Here's the drawing with two shaded views (mm, measured from the low corner). I have some questions. Coordinates: 2 decimals unless noted, no trailing zeros. Order: outer loops, then holes, each group sorted by start corner. A loop starts at its lowest first (then second) coordinate and runs counter-clockwise, first axis right, second up. Notation, with made-up numbers: (-1, 79.5) - (34, 79.5) arc R15 cw to (34, 91.5) - close; hole circle Ø5 at (73.25, 42). An arc over 180 degrees is marked (long way). Answer as a JSON object with one key per item and string values. Group by question number.
(1) Will these pins go through, and if not, where does the flat tip stop? P1, Ø0.9, axis at y = 5.5, z = 2, coming from the +X side; P2, Ø0.9, axis at x = 2, z = 1, coming from the -Y side; P3, Ø1.5, axis at y = 9.5, z = 1, coming from the -X side.
(2) Please list where these lines run through material, in increasing order: probe 1 along X at (y, z) = (49, 1.2); probe 2 along Y at (x, z) = (40, 0.3).
(3) Imagine slicing it at B-B, the plane y = 49.5. Write out the boundary of the cut face in (x, z).
(4) Imagine slicing it at A-A, the plane x = 100. Write out the boundary of the cut face in (y, z).
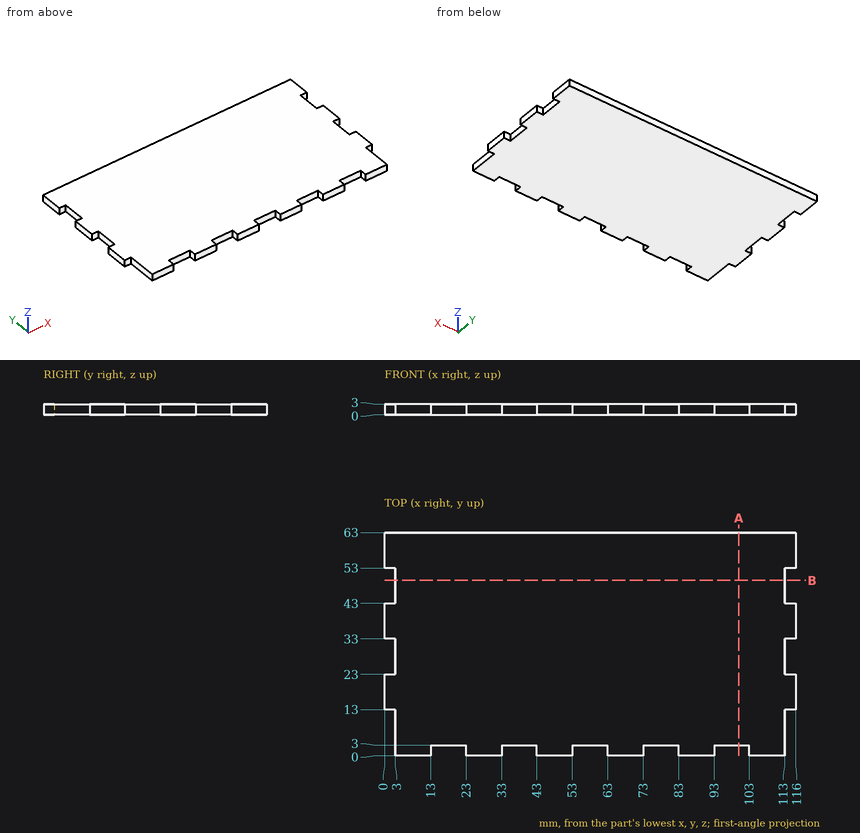
Result set:
{
 "1": {"P1": "stops at x = 113", "P2": "stops at y = 13", "P3": "stops at x = 3"},
 "2": {"probe 1": "x = 3 to 113", "probe 2": "y = 3 to 63"},
 "3": {"outline": "(3, 0) - (113, 0) - (113, 3) - (3, 3) - close"},
 "4": {"outline": "(3, 0) - (63, 0) - (63, 3) - (3, 3) - close"}
}
